Autodesk Fusion 360 part; units mm, degrees
sketch "Sketch1" plane through (0, 0, 0) normal (0, 0, 1) x (1, 0, 0)
  circle A0 centre (0, 0) radius 4
  circle A1 centre (0, 0) radius 11
  circle A2 centre (0, 0) radius 13.5
  circle A3 centre (0, 36) radius 9
  line L0 (0, 0) -> (0, 45)
  line L1 (-3.7528, 42.5) -> (-7.5056, 36)
  line L2 (-7.5056, 36) -> (-3.7528, 29.5)
  line L3 (-3.7528, 29.5) -> (3.7528, 29.5)
  line L4 (3.7528, 29.5) -> (7.5056, 36)
  line L5 (7.5056, 36) -> (3.7528, 42.5)
  line L6 (3.7528, 42.5) -> (-3.7528, 42.5)
  line L7 (9, 36) -> (13.3906, 1.7148)
  line L8 (-9, 36) -> (-13.3906, 1.7148)
  line L9 (-26.6769, -25.7942) -> (5.2102, -12.4541)
  circle A4 centre (-31.1769, -18) radius 9
  line L10 (-27.4241, -24.5) -> (-23.6714, -18)
  line L11 (-34.9297, -24.5) -> (-27.4241, -24.5)
  line L12 (-38.6825, -18) -> (-34.9297, -24.5)
  line L13 (-27.4241, -11.5) -> (-34.9297, -11.5)
  line L14 (-23.6714, -18) -> (-27.4241, -11.5)
  line L15 (-34.9297, -11.5) -> (-38.6825, -18)
  line L16 (-35.6769, -10.2058) -> (-8.1804, 10.7392)
  line L17 (35.6769, -10.2058) -> (8.1804, 10.7392)
  circle A5 centre (31.1769, -18) radius 9
  line L18 (34.9297, -11.5) -> (27.4241, -11.5)
  line L19 (38.6825, -18) -> (34.9297, -11.5)
  line L20 (34.9297, -24.5) -> (38.6825, -18)
  line L21 (23.6714, -18) -> (27.4241, -24.5)
  line L22 (27.4241, -11.5) -> (23.6714, -18)
  line L23 (27.4241, -24.5) -> (34.9297, -24.5)
  line L24 (26.6769, -25.7942) -> (-5.2102, -12.4541)
  point P0 (0, 36)
  point P1 (0, 36)
  point P2 (0, 36)
  point P3 (0, 36)
  point P4 (0, 36)
  dimension "d1" = 8
  dimension "d2" = 22
  dimension "d3" = 27
  dimension "d10" = 18
  dimension "d12" = 6.5
  dimension "d14" = 360
extrude "Extrude1" add sketch "Sketch1" along normal blind 8 contours A2 | A2 A3 L0 L8 L16 | A2 A3 L0 L7 L17 | A2 L7 L17 | A2 L8 L16 | A3 L0 L3 L4 L5 L6 | A3 L0 L1 L2 L3 L6 | A2 L7 L9 L17 A5 L24 | A2 L8 L9 A4 L16 L24 | A5 | A2 L9 L24 | A4
Input: part model. Units: mm. Frame: model coordinates. A direction names the side the tool comes from. Round coordinates to 2 decimals unless told otherwise and drop trailing zeros. Write each loop counter-clockwise with the first axis right and the second up, starting at its lowest first coordinate (ties: lowest second). Pieces come first, ordered by that corner, then holes.
1) Cut plane B-B (x = 29.5). Return the cut outline in (y, z).
2) Cut plane A-A (y = 10). Return the cut outline in (x, z), then the cut area to 3 significant figures.
3) Contact query for flat-ended pins moving along their axis: P1, Ø1, axis at y = 16, z = 1, coming from the -X side; P2, Ø4, axis at x = 31.5, z = 5.5, coming from the +Y side; P3, Ø2.5, axis at x = -1.5, z = 2.5, coming from the -Y side. Output: stop coordinate, or through.
4) Cut plane C-C (z = 3.5). Return the cut outline in (x, y).
5) Cut plane D-D (x = -2). Return the cut outline in (y, z), then the cut area to 3 significant figures.
6) Draft query along Y for faces 3 (the flat face through (-13.525, -20.292, 3.944)), 4 (the cylindrical face through (-2.38, 10.74, 3.94)), 5 (the flat face through (-9, -7, 8)). Return one class per face: pulls with the +Y half, pulls with the -Y half, needs draft (parallel to the pull), parting line crosses it, or undercut.
7) Reachability of faces 1 (the flat face through (-10.81, 21.86, 3.94)), 2 (the flat face through (-25.52, -14.8, 3.94)) from +Z, -Z, +X, -X, +Y, -Y: full face, straight path, thin tool, end or side. Return the list, or none.
Geometry says:
1. outline: (-26.84, 0) - (-24.5, 0) - (-24.5, 8) - (-26.84, 8) - close; (-11.5, 0) - (-5.5, 0) - (-5.5, 8) - (-11.5, 8) - close
2. outline: (-12.33, 0) - (-4.58, 0) - (-4.58, 8) - (-12.33, 8) - close; (4.58, 0) - (12.33, 0) - (12.33, 8) - (4.58, 8) - close
2. area: 124 mm2
3. P1: stops at x = -11.63
3. P2: stops at y = -5.5
3. P3: stops at y = -15.78
4. outline: (-35.68, -10.21) arc R9 ccw to (-26.68, -25.79) - (0, -14.63) - (26.68, -25.79) arc R9 ccw to (35.68, -10.21) - (12.67, 7.32) - (9, 36) arc R9 ccw to (-9, 36) - (-12.67, 7.32) - close; hole (-38.68, -18) - (-34.93, -24.5) - (-27.42, -24.5) - (-23.67, -18) - (-27.42, -11.5) - (-34.93, -11.5) - close; hole circle Ø22 at (0, 0); hole (-7.51, 36) - (-3.75, 29.5) - (3.75, 29.5) - (7.51, 36) - (3.75, 42.5) - (-3.75, 42.5) - close; hole (23.67, -18) - (27.42, -24.5) - (34.93, -24.5) - (38.68, -18) - (34.93, -11.5) - (27.42, -11.5) - close
5. outline: (-15.47, 0) - (-10.82, 0) - (-10.82, 8) - (-15.47, 8) - close; (10.82, 0) - (29.5, 0) - (29.5, 8) - (10.82, 8) - close; (42.5, 0) - (44.77, 0) - (44.77, 8) - (42.5, 8) - close
5. area: 205 mm2
6. face 3: pulls with the -Y half
6. face 4: undercut
6. face 5: needs draft
7. face 1: +Z, -Z, -X, +Y
7. face 2: +Z, -Z
